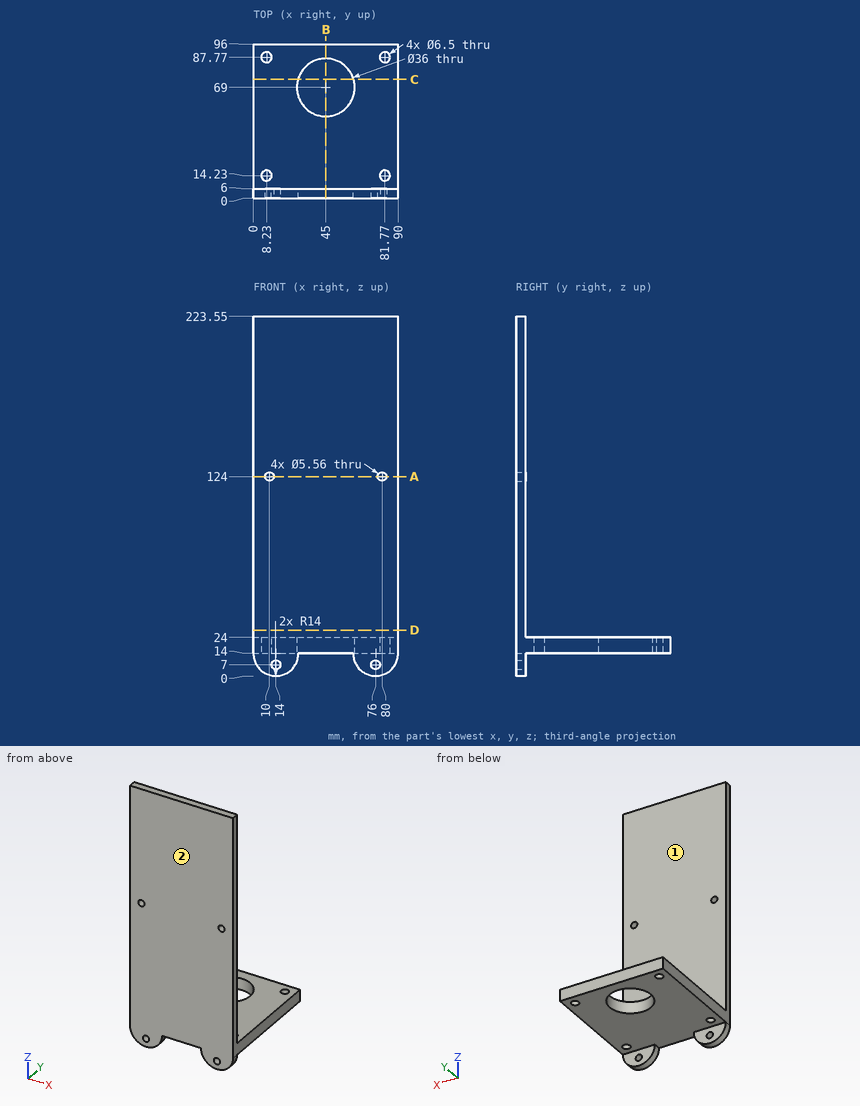
Check sheet for the drawn part. Datum: minimum x, y, z corner. Units: mm. A direction names the side the tool comes from. Give positions to 0.01 mm unless a question says otherwise; leave off trailing zeros. Loops run counter-clockwise (first coordinate to the right, second up) from the corner with the lowest first, then second, coordinate; pieces in that order, holes last. Notation, with made-up numbers: (19, 35) - (39, 35) arc R17 cw to (39, 60) - close; hole circle Ø7 at (21.25, 8). An arc over 180 degrees is marked (long way). Write each question's results on one line, items separated by ' | '.
1) Material ranges on L1, parallel to Y at x = 46, z = 195; L2, parallel to Z at x = 62, y = 15; L3, parallel to Y at x = 52.5, z = 21, recorded low to high. Write a range as from..to.
Solution:
L1: 0..6 | L2: 14..24 | L3: 0..52.64, 85.36..96
2) Sectioned sample at D-D on z = 28.5. Record the boundary of the cut face in (x, y), plus the area to 3 significant figures.
Solution:
outline: (0, 0) - (90, 0) - (90, 6) - (0, 6) - close | area: 540 mm2
3) Sectioned sample at A-A on z = 124. Record the boundary of the cut face in (x, y).
Solution:
outline: (0, 0) - (7.22, 0) - (7.22, 6) - (0, 6) - close; (12.78, 0) - (77.22, 0) - (77.22, 6) - (12.78, 6) - close; (82.78, 0) - (90, 0) - (90, 6) - (82.78, 6) - close
4) Tool access check on the marked faces 1 and 2. Record the directions out of +Z, -Z, +X, -X, +Y, -Y that give a thin tool (end or side, any length) a straight path to the whole face; none if there is none.
Solution:
face 1: +Z, +X, -X, +Y | face 2: +Z, -Z, +X, -X, -Y
5) Sectioned sample at B-B on x = 45. Record the boundary of the cut face in (y, z), plus the area to 3 significant figures.
Solution:
outline: (0, 14) - (51, 14) - (51, 24) - (6, 24) - (6, 223.55) - (0, 223.55) - close; (87, 14) - (96, 14) - (96, 24) - (87, 24) - close | area: 1,800 mm2
6) Sectioned sample at C-C on y = 74. Record the boundary of the cut face in (x, z).
Solution:
outline: (0, 14) - (27.71, 14) - (27.71, 24) - (0, 24) - close; (62.29, 14) - (90, 14) - (90, 24) - (62.29, 24) - close
7) Depth check by flat-ended pin: P1, Ø6.5, axis at x = 80, z = 124, coming from the +Y side; P2, Ø12, axis at x = 23, y = 66, coming from the +Z side; P3, Ø10.5, axis at x = 8.23, y = 87.77, coming from the -Z side. Enter the tip coordinate at first touch or a pass-through.
Solution:
P1: y = 6 | P2: z = 24 | P3: z = 14
